Input: part model. Units: mm. Frame: model coordinates. Coordinates: 2 decimals unless noted, no trailing zeros. Order: outer loops, then holes, each group sorted by start corner. A loop starts at its lowest first (then second) coordinate and runs counter-clockwise, first axis right, second up. Notation, with made-up numbers: (-11, -4.5) -> (46, -4.5) arc R19 cw to (46, 11.5) -> close; hole circle Ø4 at (64.25, 63). An arc over 180 degrees is marked (long way). One line per item, written item: value. Start each with the question number.
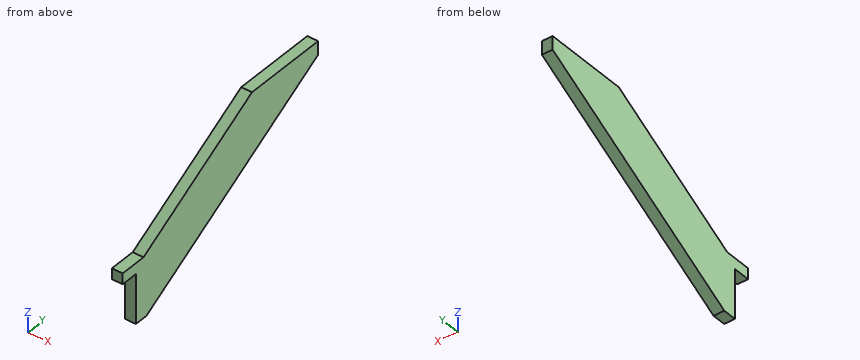
from build123d import *

# Parameters (mm, degrees)
F1_DEPTH = 40


with BuildPart() as f1:
    # F0 (on Right) → F1 (new body)
    with BuildSketch(Plane.YZ):
        Polygon((100, 182.927519083), (100, 202.0725942164), (136.1217894571, 222.927519083), (37.343967706, 222.927519083), (37.343967706, 182.927519083), align=None)
        Polygon((136.1217894571, 222.927519083), (100, 202.0725942164), (100, 182.927519083), (357.343967706, 182.927519083), (357.343967706, 222.927519083), align=None)
        Polygon((650.6664199358, 520), (136.1217894571, 222.927519083), (357.343967706, 222.927519083), (357.343967706, 182.927519083), (100, 182.927519083), (100, 0), (150, 0), (964.0638795574, 470), (964.0638795574, 520), align=None)
    extrude(amount=F1_DEPTH)


solid = f1.part
1) Ray query, line 1 along Z through (x, y) = (11, 117.5); line 2 along Y through (x, z) = (21.5, 326); line 3 along Y through (x, z) = (4, 408.5). Return the intervals inside material, ascending. Write a range as from..to.
2) Pin query (flat end, axial travel): pin 1 Ø6 at (x, y) = (11.5, 845) entering from -Z; pin 2 Ø12 at (x, z) = (21, 76.5) entering from -Y; pin 3 Ø12 at (x, y) = (33, 162) entering from -Z; pin 4 Ø10 at (y, z) = (524, 383) entering from -X. Return the tip coordinate at first contact, or that it passes through.
3) Section query B-B, the plane y = 840.5. Return the cut outline in (x, z).
4) Section query A-A, the plane x = 19. Return the cut outline in (y, z).
5) Section query C-C, the plane z = 36. Return the cut outline in (x, y).
Entries:
1. line 1: z = 0..222.93
1. line 2: y = 314.65..714.65
1. line 3: y = 457.54..857.54
2. pin 1: stops at z = 399.53
2. pin 2: stops at y = 100
2. pin 3: stops at z = 3.46
2. pin 4: stops at x = 0
3. outline: (0, 398.66) -> (40, 398.66) -> (40, 520) -> (0, 520) -> close
4. outline: (37.34, 182.93) -> (100, 182.93) -> (100, 0) -> (150, 0) -> (964.06, 470) -> (964.06, 520) -> (650.67, 520) -> (136.12, 222.93) -> (37.34, 222.93) -> close
5. outline: (0, 100) -> (40, 100) -> (40, 212.35) -> (0, 212.35) -> close
